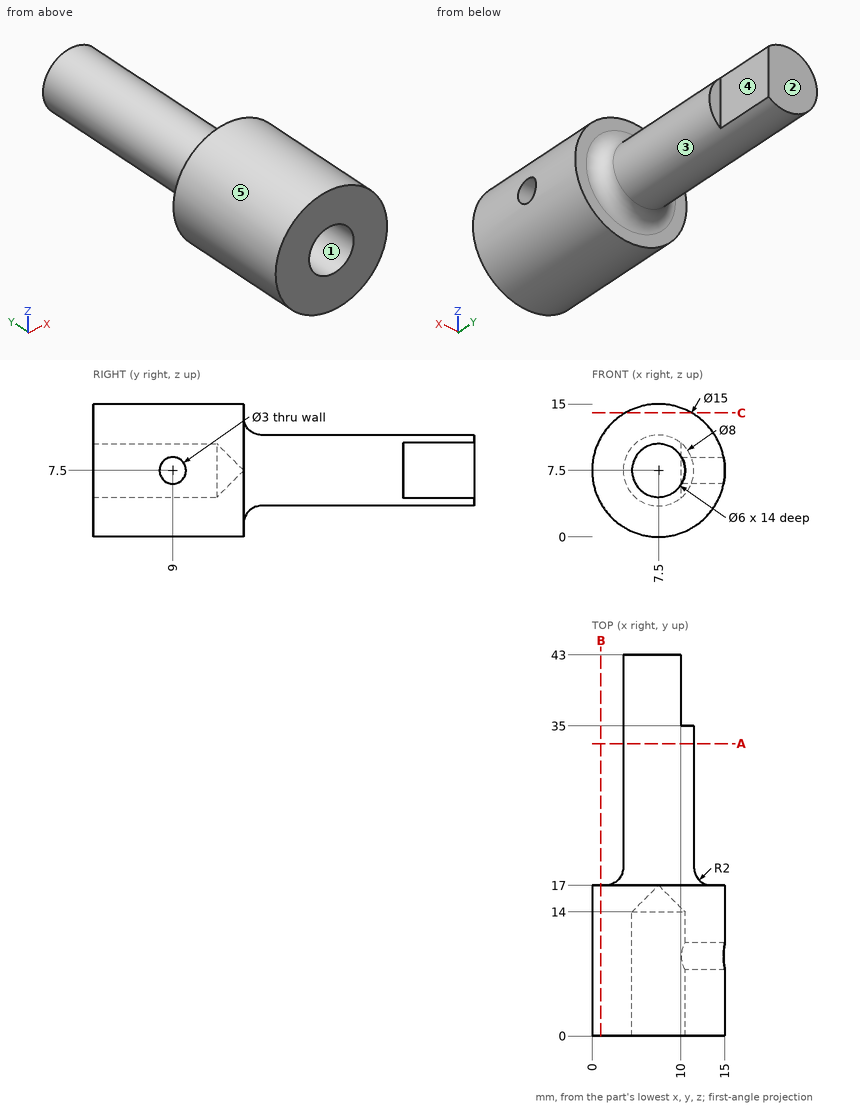
Verification items for this drawing (mm, ordinates from the low corner). A direction names the side the tool comes from. Coordinates: 2 decimals unless noted, no trailing zeros. Write each loop counter-clockwise with the first axis right and the second up, starting at its lowest first coordinate (ties: lowest second). Pieces come first, ordered by that corner, then holes. Notation, with made-up numbers: M -4,25.5 L 24,25.5 A21 cw 24,61.5 Z; hole C 5,7 d10. An arc over 180 degrees is marked long. Answer as a JSON object with one key per item and string values. Group by question number.
(1) Cross-section at A-A, the plane y = 33. Record the cut outline in (x, z).
(2) Gauge pin test, flat ends, axial feed: pin 1 (5 mm diameter, centred on y = 39.5, z = 7, fed in from +X); pin 2 (5 mm diameter, centred on x = 2.5, y = 28.5, fed in from -Z); pin 3 (2 mm diameter, centred on x = 11.5, y = 22.5, fed in from -Z). Record the tip position at first contact, or that the pin passes through.
(3) Material ranges on line 1 (Z direction, x = 7.5, y = 11.25); line 2 (Y direction, x = 10.5, z = 13); line 3 (Z direction, x = 5.75, y = 11), recorded low to high.
(4) Cross-section at C-C, the plane z = 14. Record the cut outline in (x, y).
(5) Tool access check on the marked faces 4 and 5. Record the directions out of +Z, -Z, +X, -X, +Y, -Y that give a thin tool (end or side, any length) a straight path to the whole face; none if there is none.
(6) Release check for a two-part mould opening along X. For the marked faces 1, 2 and 3 record: +X half, -X half, draft (parallel to the pull), parting line (faces both ways), or undercut.
(7) Cross-section at B-B, the plane x = 1. Record the cut outline in (y, z), and give its area (3 significant figures).
Reply:
{
 "1": {"outline": "C 7.5,7.5 d8"},
 "2": {"pin 1": "x = 10", "pin 2": "z = 4.38", "pin 3": "z = 4.85"},
 "3": {"line 1": "0 to 4.5, 10.5 to 15", "line 2": "0 to 17", "line 3": "0.21 to 5.06, 9.94 to 14.79"},
 "4": {"outline": "M 3.76,0 L 11.24,0 L 11.24,17 L 3.76,17 Z"},
 "5": {"face 4": "+Z, -Z, +X, +Y", "face 5": "+Y, -Y"},
 "6": {"face 1": "undercut", "face 2": "draft", "face 3": "parting line"},
 "7": {"outline": "M 0,3.76 L 17,3.76 L 17,11.24 L 0,11.24 Z", "area": "127 mm²"}
}
